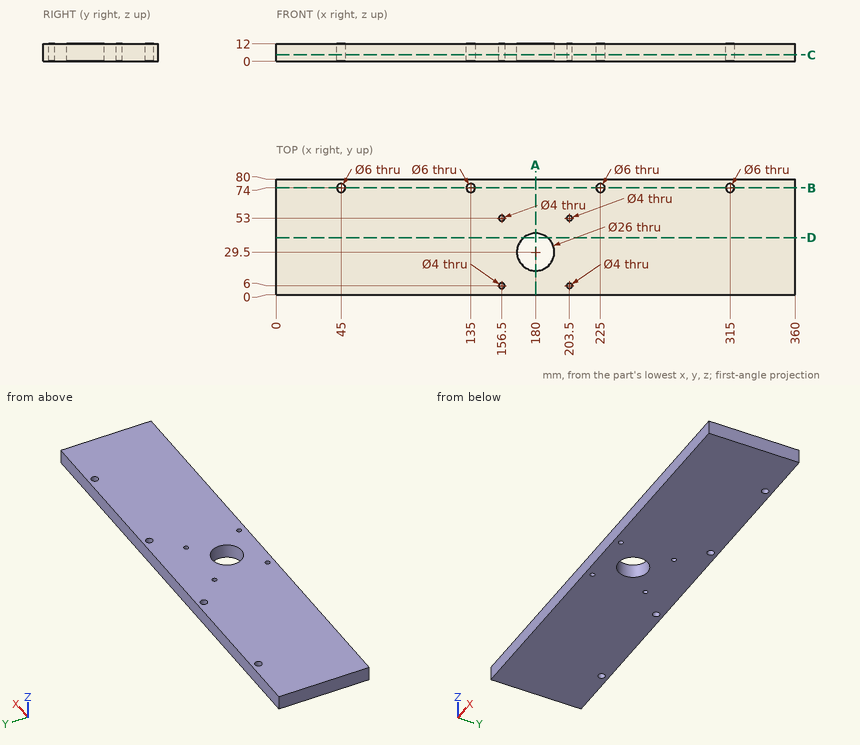
Print and shaded views of the part. All mm, measured from the part's lowest x, y and z. Give positions to 0.01 mm unless a question says otherwise; leave off trailing zeros. Loops run counter-clockwise (first coordinate to the right, second up) from the corner with the lowest first, then second, coordinate; pieces in that order, holes last.
1) Saw through at A-A (x = 180). Write the cut outline in (y, z).
2) Wall check: line 1 (Y direction, x = 203.5, z = 7.5); line 2 (Y direction, x = 225, z = 8.75); line 3 (X direction, y = 75, z = 6.75). Give the ranges that are in metal, low to high.
3) Saw through at C-C (z = 4.5). Count the separate pieces of the cut face and the enclosed holes in it, plus the area to 3 significant figures.
4) Saw through at B-B (y = 74). Write the cut outline in (x, z).
5) Saw through at D-D (y = 39.5). Write the cut outline in (x, z), plus the area to 3 significant figures.
6) Flat gauge pin, fed straight in: pin 1 Ø9.5 at (x, y) = (45, 74) entering from +Z. Where does the tip first touch, or does it go through?
Answer block:
1. outline: (0, 0) - (16.5, 0) - (16.5, 12) - (0, 12) - close; (42.5, 0) - (80, 0) - (80, 12) - (42.5, 12) - close
2. line 1: y = 0 to 4, 8 to 51, 55 to 80
2. line 2: y = 0 to 71, 77 to 80
2. line 3: x = 0 to 42.17, 47.83 to 132.17, 137.83 to 222.17, 227.83 to 312.17, 317.83 to 360
3. separate pieces: 1
3. enclosed holes: 9
3. area: 28,100 mm2
4. outline: (0, 0) - (42, 0) - (42, 12) - (0, 12) - close; (48, 0) - (132, 0) - (132, 12) - (48, 12) - close; (138, 0) - (222, 0) - (222, 12) - (138, 12) - close; (228, 0) - (312, 0) - (312, 12) - (228, 12) - close; (318, 0) - (360, 0) - (360, 12) - (318, 12) - close
5. outline: (0, 0) - (171.69, 0) - (171.69, 12) - (0, 12) - close; (188.31, 0) - (360, 0) - (360, 12) - (188.31, 12) - close
5. area: 4,120 mm2
6. pin 1: stops at z = 12
